from build123d import *

# Parameters (mm, degrees)
EXTRUDE_THIN1_DEPTH  = 50.8
SKETCH2_R            = 11
CUT_EXTRUDE1_DEPTH   = 90.858670283
M3_CLEARANCE_HOLE1_D = 3.6


with BuildPart() as part:
    # Sketch1 → Extrude-Thin1 (new body)
    with BuildSketch(Plane.XY):
        Polygon((0, 50.8), (0, 0), (50.8, 0), (50.8, -3.175), (-3.175, -3.175), (-3.175, 50.8), align=None)
    extrude(amount=EXTRUDE_THIN1_DEPTH)

    # Sketch2 → Cut-Extrude1 (cut, through all)
    with BuildSketch(Plane.ZY.offset(3.175)):
        with Locations((25.4, 23.8125)):
            Circle(SKETCH2_R)
    extrude(amount=-CUT_EXTRUDE1_DEPTH, mode=Mode.SUBTRACT)

    # M3 Clearance Hole1 (through all)
    with Locations(Plane.ZY.offset(3.175)):
        with Locations((9.909058191, 39.303441809), (40.890941809, 39.303441809), (40.890941809, 8.321558191), (9.909058191, 8.321558191)):
            Hole(M3_CLEARANCE_HOLE1_D / 2)


solid = part.part
Could you check a few things on this model? Use its own coordinates, in mm. A direction names the side the tool comes from. Coordinates: 2 decimals unless noted, no trailing zeros. Order: outer loops, then holes, each group sorted by start corner. A loop starts at its lowest first (then second) coordinate and runs counter-clockwise, first axis right, second up. Notation, with made-up numbers: (34, -25.75) -> (47, -25.75) arc R21 cw to (47, -6.75) -> close; hole circle Ø7 at (69, 25). An arc over 180 degrees is marked (long way). One line per question, with ' | ' between items.
Q1. On a 3-axis mill with a long thin cutter (end or side, diameter ignored), from which of +Z, -Z, +X, -X, +Y, -Y can I reach the whole of each face in a straight line? I mean faces 1 (the face through (50.8, -2, 25)), 2 (the face through (0, 37, 25)). Say none if no direction works.
Return value:
face 1: +Z, -Z, +X, +Y, -Y | face 2: +Z, -Z, +X, +Y
Q2. Imagine slicing it at B-B on y = 19. Please give me the cut outline in (x, z) (3 decimals), and give its area (3 significant figures).
Return value:
outline: (-3.175, 0) -> (0, 0) -> (0, 15.509) -> (-3.175, 15.509) -> close; (-3.175, 35.291) -> (0, 35.291) -> (0, 50.8) -> (-3.175, 50.8) -> close | area: 98.5 mm²
Q3. If I drill on L1, parallel to X at y = 23.5, z = 12.5 (3 decimals); L2, parallel to Y at x = -0.85, z = 25.4 (1 decimal), over which ranges is the centre line in solid material (lowest first)?
Return value:
L1: -3.175 to 0 | L2: -3.2 to 12.8, 34.8 to 50.8
Q4. Imagine slicing it at C-C on z = 30.5. Please give me the cut outline in (x, y) (3 decimals).
Return value:
outline: (-3.175, -3.175) -> (50.8, -3.175) -> (50.8, 0) -> (0, 0) -> (0, 14.066) -> (-3.175, 14.066) -> close; (-3.175, 33.559) -> (0, 33.559) -> (0, 50.8) -> (-3.175, 50.8) -> close
Q5. Thinking about a two-plate mould opening in Y: for faces 3 (the face through (-3.175, 23, 14)), 4 (the face through (-1.61, 17.12, 16.67)), 5 (the face through (-1.565, 37.546, 10.299)), 6 (the face through (25, 0, 25)), which applies, pulls with the +Y half, pulls with the -Y half, needs draft (parallel to the pull), parting line crosses it, or undercut?
Return value:
face 3: needs draft | face 4: undercut | face 5: undercut | face 6: pulls with the +Y half
Q6. Imagine slicing it at D-D on x = 38.5. Please give me the cut outline in (y, z) (3 decimals), and give its area (3 significant figures).
Return value:
outline: (-3.175, 0) -> (0, 0) -> (0, 50.8) -> (-3.175, 50.8) -> close | area: 161 mm²
Q7. I'm going to push flat-ended pins straight in: P1, Ø2, axis at x = 11.5, z = 32.5, coming from the +Y side; P2, Ø5, axis at y = 25, z = 15, coming from the +X side. Where does each tip first touch, or does it pass through?
Return value:
P1: y = 0 | P2: x = 0
Q8. Imagine slicing it at A-A on z = 25.4. Please give me the cut outline in (x, y) (1 decimal).
Return value:
outline: (-3.2, -3.2) -> (50.8, -3.2) -> (50.8, 0) -> (0, 0) -> (0, 12.8) -> (-3.2, 12.8) -> close; (-3.2, 34.8) -> (0, 34.8) -> (0, 50.8) -> (-3.2, 50.8) -> close
